from build123d import *

# Parameters (mm, degrees)
SKETCH1_R           = 23.99268
SKETCH1_R_2         = 1.35
BOSS_EXTRUDE1_DEPTH = 2.5
SKETCH4_R           = 3.96875
CUT_EXTRUDE3_DEPTH  = 3.5


with BuildPart() as part:
    # Sketch1 → Boss-Extrude1 (new body)
    with BuildSketch(Plane(origin=(0, 0, 0), x_dir=(1, 0, 0), z_dir=(0, 1, 0))):
        Circle(SKETCH1_R)
        with Locations((0, 11.99634)):
            Circle(SKETCH1_R_2, mode=Mode.SUBTRACT)
        with Locations((10.389135192, -5.99817)):
            Circle(SKETCH1_R_2, mode=Mode.SUBTRACT)
        with Locations((-10.389135192, -5.99817)):
            Circle(SKETCH1_R_2, mode=Mode.SUBTRACT)
    extrude(amount=BOSS_EXTRUDE1_DEPTH)

    # Sketch4 → Cut-Extrude3 (cut, through all)
    with BuildSketch(Plane(origin=(0, 2.5, 0), x_dir=(1, 0, 0), z_dir=(0, 1, 0))):
        Circle(SKETCH4_R)
    extrude(amount=-CUT_EXTRUDE3_DEPTH, mode=Mode.SUBTRACT)


solid = part.part
CAD build for the part. Positions are in the model's coordinates, mm. Coordinates: 2 decimals unless noted, no trailing zeros. Write each loop counter-clockwise with the first axis right and the second up, starting at its lowest first coordinate (ties: lowest second). Pieces come first, ordered by that corner, then holes. Notation, with made-up numbers: (-15, 8) - (-6, 8) arc R27 cw to (-6, 35) - close; hole circle Ø9 at (12, 77). An arc over 180 degrees is marked (long way). Use a Markdown table: item, result. Add a question column.
Item 1: Band-saw the part on D-D, the plane z = -19. Give the cut face in (x, y), and give its area (3 significant figures).
Item 2: Mould opens along Z. For faces 1 (the face through (-5.201, 1.232, 23.422)), 2 (the face through (9.32, 1.23, 6.82)), 3 (the face through (-0.293, 1.232, -10.678)), 4 (the face through (0, 0, 5)) say: pulls with the +Z half, pulls with the -Z half, needs draft (parallel to the pull), parting line crosses it, or undercut.
Item 3: Flat gauge pins, fed straight in: pin 1 (1 mm diameter, centred on y = 2, z = 13.5, fed in from -X); pin 2 (1 mm diameter, centred on x = -3, y = 2, fed in from +Z). Where does each tip first touch, or does it go through?
Item 4: Band-saw the part on C-C, the plane y = 1. Give the cut face in (x, z).
Item 5: Band-saw the part on B-B, the plane z = 0. Give the cut face in (x, y), and give its area (3 significant figures).
Item 6: Band-saw the part on A-A, the plane x = 0. Give the cut face in (y, z), and give its area (3 significant figures).
Item 7: Drill centre lines: L1, parallel to Z at x = 0, y = 0.5; L2, parallel to X at y = 0.9, z = 0; L3, parallel to X at y = 0.4, z = 6. Where is each one in solid material? Low to high. Write a range as from..to.
Numbers:
| question | item | result |
|---|---|---|
| 1 | outline | (-14.65, 0) - (14.65, 0) - (14.65, 2.5) - (-14.65, 2.5) - close |
| 1 | area | 73.3 mm2 |
| 2 | face 1 | parting line crosses it |
| 2 | face 2 | undercut |
| 2 | face 3 | undercut |
| 2 | face 4 | needs draft |
| 3 | pin 1 | x = -20.17 |
| 3 | pin 2 | z = 23.86 |
| 4 | outline | circle Ø47.99 at (0, 0); hole circle Ø2.7 at (-10.39, 6); hole circle Ø7.94 at (0, 0); hole circle Ø2.7 at (0, -12); hole circle Ø2.7 at (10.39, 6) |
| 5 | outline | (-23.99, 0) - (-3.97, 0) - (-3.97, 2.5) - (-23.99, 2.5) - close; (3.97, 0) - (23.99, 0) - (23.99, 2.5) - (3.97, 2.5) - close |
| 5 | area | 100 mm2 |
| 6 | outline | (0, -23.99) - (2.5, -23.99) - (2.5, -13.35) - (0, -13.35) - close; (0, -10.65) - (2.5, -10.65) - (2.5, -3.97) - (0, -3.97) - close; (0, 3.97) - (2.5, 3.97) - (2.5, 23.99) - (0, 23.99) - close |
| 6 | area | 93.4 mm2 |
| 7 | L1 | -23.99..-13.35, -10.65..-3.97, 3.97..23.99 |
| 7 | L2 | -23.99..-3.97, 3.97..23.99 |
| 7 | L3 | -23.23..-11.74, -9.04..9.04, 11.74..23.23 |
